Design review of the part shown in the three views and the two pictorial views. Dimensions are in mm from the part's minimum x, y and z. A direction names the side the tool comes from. Round coordinates to 2 decimals unless told otherwise and drop trailing zeros. Order: outer loops, then holes, each group sorted by start corner. A loop starts at its lowest first (then second) coordinate and runs counter-clockwise, first axis right, second up.
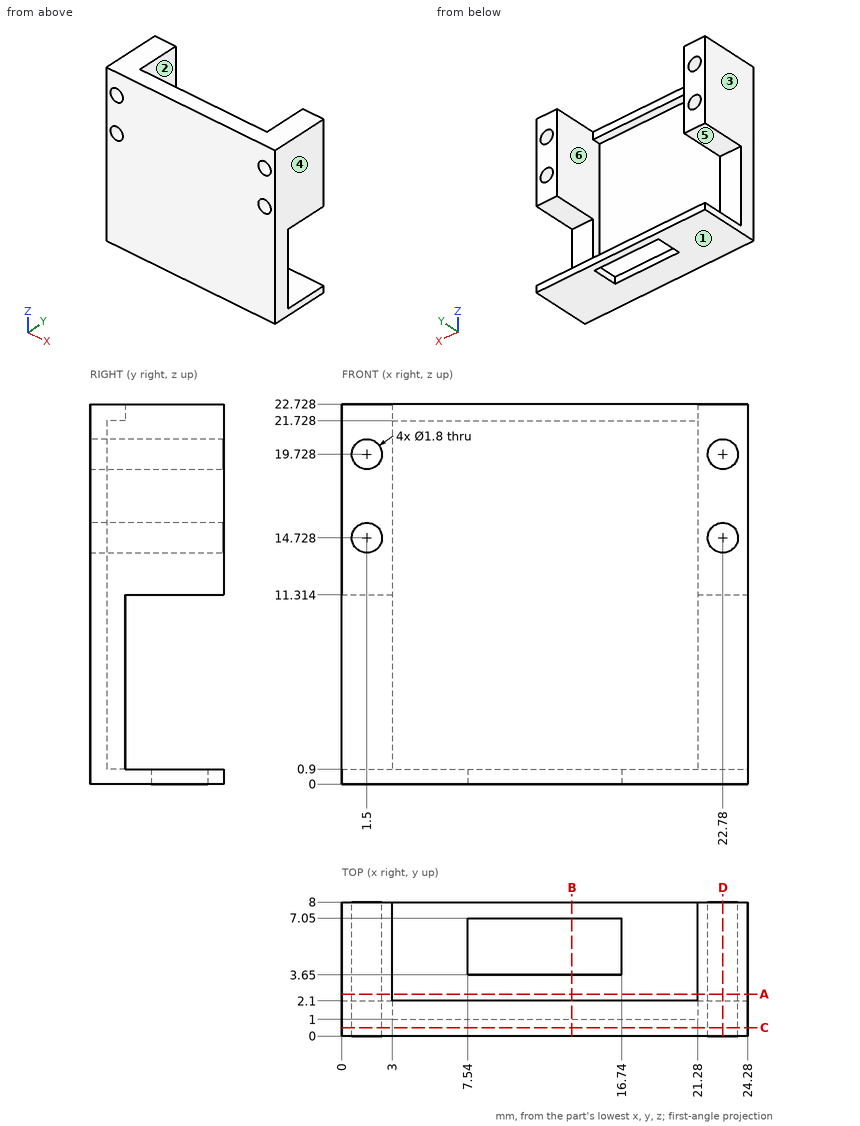
1) For the marked faces 4, 5 and 6, list the 3-axis set-ups (+Z, -Z, +X, -X, +Y, -Y) from which the entire face can be reached by the end or side of a thin tool; tool diameter is ignored.
Results:
face 4: +Z, -Z, +X, +Y, -Y
face 5: +X, -X, +Y
face 6: +Y
2) The part is to be moulded in two halves that separate along X. For the marked faces 1, 2 and 3, say which applies: released by +X, released by -X, zero draft, split by the parting line, or undercut.
Results:
face 1: zero draft
face 2: undercut
face 3: released by -X
3) Clearance check with flat-ended pins moving along their axes: P1, Ø3.5, axis at x = 23, z = 7, coming from the +Y side; P2, Ø1.4, axis at x = 22.78, z = 14.728, coming from the -Y side; P3, Ø5.5, axis at x = 11.5, z = 10.5, coming from the +Y side. State where each tip first meets the part, or that it passes through.
Results:
P1: stops at y = 2.1
P2: passes through
P3: stops at y = 1
4) Take a section at C-C on y = 0.5. Give the boundary of the cut face in (x, z).
Results:
outline: (0, 0) - (24.28, 0) - (24.28, 22.73) - (0, 22.73) - close; hole circle Ø1.8 at (1.5, 14.73); hole circle Ø1.8 at (1.5, 19.73); hole circle Ø1.8 at (22.78, 14.73); hole circle Ø1.8 at (22.78, 19.73)
5) Take a section at B-B on x = 13.75. Give the boundary of the cut face in (y, z), plus the area to 3 significant figures.
Results:
outline: (0, 0) - (3.65, 0) - (3.65, 0.9) - (1, 0.9) - (1, 21.73) - (2.1, 21.73) - (2.1, 22.73) - (0, 22.73) - close; (7.05, 0) - (8, 0) - (8, 0.9) - (7.05, 0.9) - close
area: 27.1 mm2
6) To check wall thickness, follow line 1 along X through (y, z) = (3.5, 13.25); line 2 along X through (y, z) = (5.5, 19); line 3 along Y through (x, z) = (21, 17.5). State the ranges of each line that lie inside material, in increasing order.
Results:
line 1: x = 0 to 3, 21.28 to 24.28
line 2: x = 0 to 0.97, 2.03 to 3, 21.28 to 22.25, 23.31 to 24.28
line 3: y = 0 to 1
7) Take a section at D-D on x = 22.78. Give the boundary of the cut face in (y, z), plus the area to 3 significant figures.
Results:
outline: (0, 0) - (8, 0) - (8, 0.9) - (2.1, 0.9) - (2.1, 11.31) - (8, 11.31) - (8, 13.83) - (0, 13.83) - close; (0, 15.63) - (8, 15.63) - (8, 18.83) - (0, 18.83) - close; (0, 20.63) - (8, 20.63) - (8, 22.73) - (0, 22.73) - close
area: 91.6 mm2
8) Take a section at A-A on y = 2.5. Give the boundary of the cut face in (x, z), plus the area to 3 significant figures.
Results:
outline: (0, 0) - (24.28, 0) - (24.28, 0.9) - (0, 0.9) - close; (0, 11.31) - (3, 11.31) - (3, 22.73) - (0, 22.73) - close; (21.28, 11.31) - (24.28, 11.31) - (24.28, 22.73) - (21.28, 22.73) - close; hole circle Ø1.8 at (1.5, 14.73); hole circle Ø1.8 at (1.5, 19.73); hole circle Ø1.8 at (22.78, 14.73); hole circle Ø1.8 at (22.78, 19.73)
area: 80.2 mm2
